Job drawing, mm, ordinate dimensions from the low corner. One solid piece. Round coordinates to 2 decimals unless told otherwise and drop trailing zeros. Loops run counter-clockwise (first coordinate to the right, second up) from the corner with the lowest first, then second, coordinate; pieces in that order, holes last.
1) Drop flat-ended pins along their axis: P1, Ø1.5, axis at y = 39.5, z = 8.5, coming from the -X side; P2, Ø5, axis at x = 240, z = 3.5, coming from the -Y side. Give the stop position or say it passes through.
2) Band-saw the part on C-C, the plane x = 25.5. Write the cut outline in (y, z), then the cut area to 3 significant figures.
3) Band-saw the part on A-A, the plane y = 24. Write the cut outline in (x, z) (1 decimal).
4) Band-saw the part on B-B, the plane z = 5.5. Write the cut outline in (x, y) (1 decimal), then the cut area to 3 significant figures.
5) Band-saw the part on D-D, the plane x = 196.5. Write the cut outline in (y, z), then the cut area to 3 significant figures.
6) Probe line 1 (X direction, y = 37, z = 8) (1 decimal); line 2 (X direction, y = 9.5, z = 4) (1 decimal); line 3 (Y direction, x = 228, z = 7.25). List the from-to ranges inside material, lowest first.
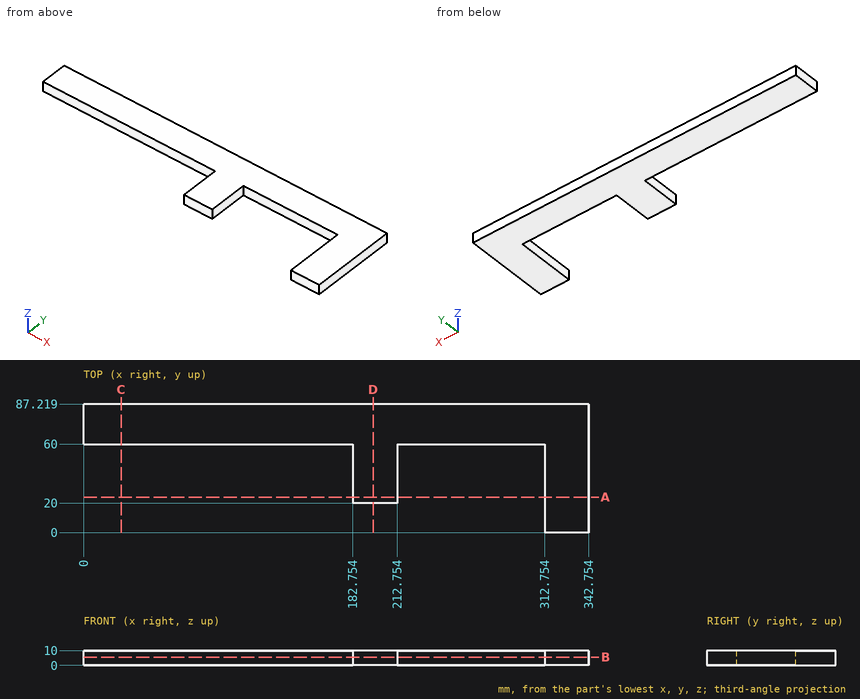
Reported:
1. P1: stops at x = 182.75
1. P2: stops at y = 60
2. outline: (60, 0) - (87.22, 0) - (87.22, 10) - (60, 10) - close
2. area: 272 mm2
3. outline: (182.8, 0) - (212.8, 0) - (212.8, 10) - (182.8, 10) - close; (312.8, 0) - (342.8, 0) - (342.8, 10) - (312.8, 10) - close
4. outline: (0, 60) - (182.8, 60) - (182.8, 20) - (212.8, 20) - (212.8, 60) - (312.8, 60) - (312.8, 0) - (342.8, 0) - (342.8, 87.2) - (0, 87.2) - close
4. area: 12,300 mm2
5. outline: (20, 0) - (87.22, 0) - (87.22, 10) - (20, 10) - close
5. area: 672 mm2
6. line 1: x = 182.8 to 212.8, 312.8 to 342.8
6. line 2: x = 312.8 to 342.8
6. line 3: y = 60 to 87.22
